Design review of the part built by this model. Coordinates are the model's own, in mm. A direction names the side the tool comes from. Coordinates: 2 decimals unless noted, no trailing zeros. Loops run counter-clockwise (first coordinate to the right, second up) from the corner with the lowest first, then second, coordinate; pieces in that order, holes last.
Q1. Add section C-C on z = 0. Give the boundary of the cut face in (x, y).
Q2. Add section B-B on y = 0. Give the boundary of the cut face in (x, z), and give its area (3 significant figures).
Q3. Add section D-D on x = -13.5. Give the boundary of the cut face in (y, z).
Q4. Machinability: for faces 1 (the face through (-10.16, -32.21, 0.04)), 2 (the face through (-6.8, -35.56, -4.5)), which of the approach directions +Z, -Z, +X, -X, +Y, -Y give a long, thin tool a straight path to every point of the face, cutting with its end or side? Answer none if there is none.
Q5. Draft analysis for pull direction X (two halves, no side actions). For faces 3 (the face through (9.69, -34.27, 3.05)), 4 (the face through (0, -38.1, 0)), 5 (the face through (1.312, 32.994, 0.036)), state which applies: released by +X, released by -X, zero draft, split by the parting line, or undercut.
Q6. For P1, Ø5, axis at y = 11, z = -4, coming from the +X side; P2, Ø4, axis at x = 5, z = -7.5, coming from the +Y side; P3, Ø12, axis at x = -7.5, z = 2, coming from the +Y side, all flat-tipped, find the tip position at first contact; note any pin that passes through.
Q7. Add section A-A on x = 0. Give the boundary of the cut face in (y, z).
Q8. Wall thickness on probe 1 along X at (y, z) = (0, 0.1); probe 2 along Y at (x, z) = (0, 0.9); probe 3 along X at (y, z) = (1.5, 0): over which ranges is each line inside the solid? List them lowest first.
```python
from build123d import *

# Parameters (mm, degrees)
F0_R     = 35.56
F0_R_2   = 33.02
F1_DEPTH = 2.54
F2_DEPTH = 2.54
F3_R     = 10.16
F4_DEPTH = 35.56
F5_DEPTH = 33.02
F6_R     = 7.94208
F7_DEPTH = 2.54


with BuildPart() as f1:
    # F0 (on Top) → F1 (new body)
    with BuildSketch(Plane.XY):
        Circle(F0_R)
        Circle(F0_R_2, mode=Mode.SUBTRACT)
    extrude(amount=F1_DEPTH)

    # F0 (on Top) → F2 (join)
    with BuildSketch(Plane.XY):
        Circle(F0_R)
        Circle(F0_R_2, mode=Mode.SUBTRACT)
    extrude(amount=-F2_DEPTH)

    # F3 (on Front) → F4 (join)
    with BuildSketch(Plane.XZ):
        Circle(F3_R)
    extrude(amount=F4_DEPTH)

    # F3 (on Front) → F5 (cut)
    with BuildSketch(Plane.XZ):
        Circle(F3_R)
    extrude(amount=F5_DEPTH, mode=Mode.SUBTRACT)

    # F6 (on face) → F7 (join)
    with BuildSketch(Plane.XZ.offset(35.56)):
        Circle(F6_R)
    extrude(amount=F7_DEPTH)


solid = f1.part
```
Entries:
1. outline: (-10.16, -35.56) - (-7.94, -35.56) - (-7.94, -38.1) - (7.94, -38.1) - (7.94, -35.56) - (10.16, -35.56) - (10.16, -34.08) arc R35.56 ccw (long way) to (-10.16, -34.08) - close; hole (-10.16, -33.02) - (10.16, -33.02) - (10.16, -31.42) arc R33.02 ccw (long way) to (-10.16, -31.42) - close
2. outline: (-35.56, -2.54) - (-33.02, -2.54) - (-33.02, 2.54) - (-35.56, 2.54) - close; (33.02, -2.54) - (35.56, -2.54) - (35.56, 2.54) - (33.02, 2.54) - close
2. area: 25.8 mm2
3. outline: (-32.9, -2.54) - (-30.13, -2.54) - (-30.13, 2.54) - (-32.9, 2.54) - close; (30.13, -2.54) - (32.9, -2.54) - (32.9, 2.54) - (30.13, 2.54) - close
4. face 1: none
4. face 2: -Y
5. face 3: split by the parting line
5. face 4: zero draft
5. face 5: undercut
6. P1: stops at x = 34.41
6. P2: stops at y = -33.02
6. P3: stops at y = 35.53
7. outline: (-38.1, -7.94) - (-35.56, -7.94) - (-35.56, -10.16) - (-33.02, -10.16) - (-33.02, 10.16) - (-35.56, 10.16) - (-35.56, 7.94) - (-38.1, 7.94) - close; (33.02, -2.54) - (35.56, -2.54) - (35.56, 2.54) - (33.02, 2.54) - close
8. probe 1: x = -35.56 to -33.02, 33.02 to 35.56
8. probe 2: y = -38.1 to -33.02, 33.02 to 35.56
8. probe 3: x = -35.53 to -32.99, 32.99 to 35.53
